Verification items for the finished model (mm, model axes). A direction names the side the tool comes from. Coordinates: 2 decimals unless noted, no trailing zeros. Write each loop counter-clockwise with the first axis right and the second up, starting at its lowest first coordinate (ties: lowest second). Pieces come first, ordered by that corner, then holes. Notation, with made-up numbers: (40.5, 47) -> (78.5, 47) arc R7 ccw to (78.5, 59) -> close; hole circle Ø1 at (74, 20.25). An arc over 180 degrees is marked (long way). Write item = value, one per line. Start each with the question number.
(1) Mould release check, pull along Z, two halves, no side actions. Record for faces 5 (the face through (-2, 5, -12)), 6 (the face through (69.513, 4.93, -2.294)), 7 (the face through (-80, -10, 0)): released by +Z, released by -Z, zero draft, split by the parting line, or undercut.
(2) Section check C-C (x = -57). Record the cut outline in (y, z), plus the area to 3 significant figures.
(3) Section check D-D (z = 47). Record the cut outline in (x, y).
(4) Material ranges on probe 1 along Z at (x, y) = (0, 4.75); probe 2 along Y at (x, z) = (-24, -7); probe 3 along Z at (x, y) = (-58, 4.75), recorded low to high. Write a range as [from, to].
(5) Gauge pin test, flat ends, axial feed: pin 1 Ø4 at (y, z) = (-3, 5) entering from -X; pin 2 Ø3 at (y, z) = (6.5, -12.5) entering from +X; pin 3 Ø8 at (x, y) = (-57.5, 3) entering from -Z; pin 4 Ø16 at (x, z) = (0, 0) entering from -Y. Record the tip position at first contact, or that the pin passes through.
(6) Section check B-B (z = 0). Record the cut outline in (x, y), plus the area to 3 significant figures.
(7) Set-up check for faces 1 (the face through (-36.97, 4.93, 28.81)), 2 (the face through (0, 5, -13.798)), 3 (the face through (11, 10, -1)), 4 (the face through (12, 0, -1)): record each of +Z, -Z, +X, -X, +Y, -Y from which the full face is reachable in a straight line by a thin tool's end or side.
(8) Section check A-A (x = 0). Record the cut outline in (y, z).
```python
from build123d import *

# Parameters (mm, degrees)
EXTRUDE_1_DEPTH = 10
EXTRUDE_START   = 10
SKETCH_2_R      = 5
EXTRUDE_2_DEPTH = 10


with BuildPart() as part:
    # 草图1 → 凸台-拉伸1 (new body)
    with BuildSketch(Plane(origin=(0, 0, 0), x_dir=(1, 0, 0), z_dir=(0, 1, 0))):
        with BuildLine():
            Line((-80, 5), (-31.520674237, 5))
            ThreePointArc((-31.520674237, 5), (-36.841255051, 28.492771834), (-49.180194883, 49.180194883))
            ThreePointArc((-49.180194883, 49.180194883), (69.551298604, 0), (-49.180194883, -49.180194883))
            ThreePointArc((-49.180194883, -49.180194883), (-36.841255051, -28.492771834), (-31.520674237, -5))
            Line((-31.520674237, -5), (-80, -5))
            ThreePointArc((-80, -5), (-85, 0), (-80, 5))
        make_face()
        with BuildLine():
            Line((-2, 9.797958971), (-2, 13.797958971))
            Line((-2, 13.797958971), (2, 13.797958971))
            Line((2, 13.797958971), (2, 9.797958971))
            ThreePointArc((2, 9.797958971), (0, -10), (-2, 9.797958971))
        make_face(mode=Mode.SUBTRACT)
    extrude(amount=EXTRUDE_1_DEPTH)

    # 草图2 → 凸台-拉伸2 (add)
    with BuildSketch(Plane.XZ.offset(EXTRUDE_START)):
        with Locations(Location((-80, 0, 0), (0, 0, 270))):
            Circle(SKETCH_2_R)
    extrude(amount=-EXTRUDE_2_DEPTH)


solid = part.part
```
Response:
q1.face_5 = undercut
q1.face_6 = split by the parting line
q1.face_7 = zero draft
q2.outline = (0, -5) -> (10, -5) -> (10, 5) -> (0, 5) -> close
q2.area = 100 mm2
q3.outline = (-47.43, 0) -> (51.27, 0) -> (51.27, 10) -> (-47.43, 10) -> close
q4.probe_1 = [-69.55, -13.8], [10, 69.55]
q4.probe_2 = [0, 10]
q4.probe_3 = [-5, 5]
q5.pin_1 = -84
q5.pin_2 = 68.68
q5.pin_3 = -5
q5.pin_4 = through
q6.outline = (-85, -10) -> (-75, -10) -> (-75, 0) -> (-10, 0) -> (-10, 10) -> (-85, 10) -> close; (10, 0) -> (69.55, 0) -> (69.55, 10) -> (10, 10) -> close
q6.area = 1,450 mm2
q7.face_1 = -X, +Y, -Y
q7.face_2 = +Y, -Y
q7.face_3 = +Z, -Z, +X, -X, +Y
q7.face_4 = +Z, -Z, +X, -Y
q8.outline = (0, -69.55) -> (10, -69.55) -> (10, -13.8) -> (0, -13.8) -> close; (0, 10) -> (10, 10) -> (10, 69.55) -> (0, 69.55) -> close
